Autodesk Inventor part; units mm, degrees
ref_plane "YZ Plane" through (0, 0, 0) normal (1, 0, 0) x (0, 1, 0)
ref_plane "XZ Plane" through (0, 0, 0) normal (0, 1, 0) x (-1, 0, 0)
ref_plane "XY Plane" through (0, 0, 0) normal (0, 0, 1) x (1, 0, 0)
sketch "Sketch1" plane through (0, 0, 0) normal (0, 1, 0) x (-1, 0, 0)
  line L0 (7, 12) -> (10, 12)
  line L1 (-7, 12) -> (-10, 12)
  line L2 (-10, 25) -> (-10, 12)
  line L3 (10, 12) -> (10, 25)
  line L4 (-10, 25) -> (10, 25)
  line L5 (7, 0) -> (-7, 0) construction
  line L6 (-7, 12) -> (-7, 0)
  line L7 (7, 12) -> (7, 0)
  line L8 (-10, 20) -> (0, 20) construction
  line L9 (-10, 20) -> (-5, 20) construction
  line L10 (10, 20) -> (5, 20) construction
  line L11 (7, -12) -> (10, -12)
  line L12 (-7, -12) -> (-10, -12)
  line L13 (-10, -25) -> (-10, -12)
  line L14 (10, -12) -> (10, -25)
  line L15 (-10, -25) -> (10, -25)
  line L16 (-7, -12) -> (-7, 0)
  line L17 (7, -12) -> (7, 0)
  line L18 (-10, -20) -> (0, -20) construction
  line L19 (-10, -20) -> (-5, -20) construction
  line L20 (10, -20) -> (5, -20) construction
  point P0 (0, 0)
  dimension "d39" = 12
  dimension "d40" = 13
  dimension "d41" = 20
extrude "Extrusion1" add sketch "Sketch1" along normal blind 1
sketch "Sketch2" plane through (0, 1, 0) normal (0, 1, 0) x (1, 0, 0)
  line L0 (-10, -12) -> (-10, -25)
  line L1 (-10, -25) -> (-10, -12)
  line L2 (-10, -12) -> (-7, -12)
  line L3 (7, -12) -> (10, -12)
  line L4 (10, -12) -> (10, -25)
  line L5 (-7, -12) -> (-7, 12)
  line L6 (7, 12) -> (7, -12)
  line L7 (10, -25) -> (-10, -25)
  line L8 (-7, 12) -> (-10, 12)
  line L9 (-10, 12) -> (-10, 25)
  line L10 (-10, 25) -> (10, 25)
  line L11 (10, 25) -> (10, 12)
  line L12 (10, 12) -> (7, 12)
  point P0 (0, 0)
  point P1 (-10, -40)
extrude "Extrusion2" add sketch "Sketch2" along normal blind 0.2
hole "Hole3" at (-5, 0, -20) at (5, 0, -20) at (0, 0, 20) direction (0, 1, 0) diameter 1.567 end through all
properties part number "PCB-blank-20x20"
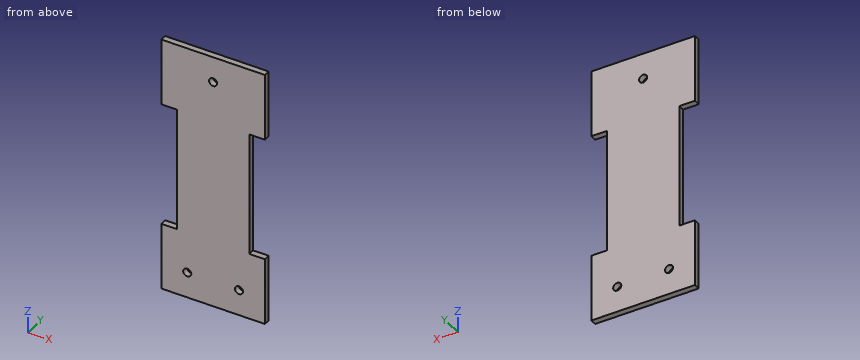
Here's how the part is built. I have some questions about the finished solid (model axes, mm). Give positions to 0.01 mm unless a question says otherwise; leave off trailing zeros. Write each loop counter-clockwise with the first axis right and the second up, starting at its lowest first coordinate (ties: lowest second). Pieces come first, ordered by that corner, then holes. Notation, with made-up numbers: M 65,-11 L 80,-11 A28 ccw 80,26 Z; hole C 9,-1.75 d9. An arc over 180 degrees is marked long. Put each result on its own line as item: value. Start each with the question number.
Item 1: Will this pin go through, and if not, where does the flat tip stop? pin 1 (0.6 mm diameter, centred on y = 1, z = -1.5, fed in from -X).
Item 2: I need wall thicknesses on L1, parallel to X at y = 0.7, z = -20; L2, parallel to Z at x = 0, y = 0.75; L3, parallel to Z at x = 5, y = 0.65. Which ranges of each line are inside material? Lowest first, please. Write a range as from..to.
Item 3: If we section it at C-C, the plane x = 0: Write out the boundary of the cut face in (y, z).
Item 4: If we section it at B-B, the plane z = 20: Write out the boundary of the cut face in (x, y).
Item 5: If we section it at D-D, the plane z = -20: Write out the boundary of the cut face in (x, y).
Item 6: If we section it at A-A, the plane y = 0.4: Write out the boundary of the cut face in (x, z), then the cut area to 3 significant figures.
Values:
1. pin 1: x = -7
2. L1: -10..-5.78, -4.22..4.22, 5.78..10
2. L2: -25..19.22, 20.78..25
2. L3: -25..-20.78, -19.22..25
3. outline: M 0,-25 L 1.2,-25 L 1.2,19.22 L 0,19.22 Z; M 0,20.78 L 1.2,20.78 L 1.2,25 L 0,25 Z
4. outline: M -10,0 L -0.78,0 L -0.78,1.2 L -10,1.2 Z; M 0.78,0 L 10,0 L 10,1.2 L 0.78,1.2 Z
5. outline: M -10,0 L -5.78,0 L -5.78,1.2 L -10,1.2 Z; M -4.22,0 L 4.22,0 L 4.22,1.2 L -4.22,1.2 Z; M 5.78,0 L 10,0 L 10,1.2 L 5.78,1.2 Z
6. outline: M -10,-25 L 10,-25 L 10,-12 L 7,-12 L 7,12 L 10,12 L 10,25 L -10,25 L -10,12 L -7,12 L -7,-12 L -10,-12 Z; hole C -5,-20 d1.57; hole C 0,20 d1.57; hole C 5,-20 d1.57
6. area: 850 mm²
